```python
from build123d import *

# Parameters (mm, degrees)
F1_DEPTH = 1000


with BuildPart() as f1:
    # F0 (on Front) → F1 (new body)
    with BuildSketch(Plane.XZ):
        with BuildLine():
            Line((-72.4, 558.240645), (-72.4, 541.240645))
            Line((-72.4, 541.240645), (82, 541.240645))
            Line((82, 541.240645), (82, 558.240645))
            Line((82, 558.240645), (19.8, 558.240645))
            ThreePointArc((19.8, 558.240645), (12.587511, 561.228156), (9.6, 568.440645))
            Line((9.6, 568.440645), (9.6, 976.040645))
            ThreePointArc((9.6, 976.040645), (12.587511, 983.253134), (19.8, 986.240645))
            Line((19.8, 986.240645), (82, 986.240645))
            Line((82, 986.240645), (82, 1003.240645))
            Line((82, 1003.240645), (-72.4, 1003.240645))
            Line((-72.4, 1003.240645), (-72.4, 986.240645))
            Line((-72.4, 986.240645), (-10.2, 986.240645))
            ThreePointArc((-10.2, 986.240645), (-2.987511, 983.253134), (0, 976.040645))
            Line((0, 976.040645), (0, 568.440645))
            ThreePointArc((0, 568.440645), (-2.987511, 561.228156), (-10.2, 558.240645))
            Line((-10.2, 558.240645), (-72.4, 558.240645))
        make_face()
    extrude(amount=-F1_DEPTH)


solid = f1.part
```
Work out the finished part from the listing and answer in its coordinate system (mm). A direction names the side the tool comes from. Give positions to 0.01 mm unless a question says otherwise; leave off trailing zeros. Order: outer loops, then holes, each group sorted by start corner. A loop starts at its lowest first (then second) coordinate and runs counter-clockwise, first axis right, second up. Notation, with made-up numbers: (-26.75, 57) -> (26.25, 57) arc R23 ccw to (26.25, 89) -> close; hole circle Ø1 at (52.25, 58.5). An arc over 180 degrees is marked (long way). Answer as CSV lines item,"result". Start each with the question number.
(1) Section C-C, the plane z = 959 is taken. Write down the section's boundary in (x, y).
(2) Consider line 1 along Z through (x, y) = (64, 953); line 2 along Z through (x, y) = (-9.5, 335.5); line 3 along X through (y, z) = (649, 893). Determine where each line is inside the solid, lowest interval first.
(3) Which of the six approach directions +Z, -Z, +X, -X, +Y, -Y give full straight-line access (tool end or side, diameter ignored) to faces 1 (the flat face through (-41, 493, 558.241)), 2 (the flat face through (51, 493, 558.241)), 3 (the flat face through (6, 493, 1003.241))?
(4) Section B-B, the plane y = 158.5 is taken. Write down the section's boundary in (x, z).
(5) For a pull along Z with two mould halves and no side action, classify faces 4 (the flat face through (-72.4, 493, 550)), 5 (the flat face through (50, 493, 986.241)), 6 (the flat face through (4, 493, 541.241)) as released by +Z, released by -Z, zero draft, split by the parting line, or undercut.
(6) Each of these flat-tipped pins is pushed along its axis until it touches: pin 1 Ø10 at (y, z) = (124, 629) entering from -X; pin 2 Ø6 at (x, z) = (3, 786.5) entering from -Y. Where does it stop, or does it pass through?
(7) Section A-A, the plane x = -22 is taken. Write down the section's boundary in (y, z), plus the area to 3 significant figures.
Entries:
1,outline,"(0, 0) -> (9.6, 0) -> (9.6, 1000) -> (0, 1000) -> close"
2,line 1,"541.24 to 558.24, 986.24 to 1003.24"
2,line 2,"541.24 to 558.26, 986.22 to 1003.24"
2,line 3,"0 to 9.6"
3,face 1,"-X, +Y, -Y"
3,face 2,"+X, +Y, -Y"
3,face 3,"+Z, +X, -X, +Y, -Y"
4,outline,"(-72.4, 541.24) -> (82, 541.24) -> (82, 558.24) -> (19.8, 558.24) arc R10.2 cw to (9.6, 568.44) -> (9.6, 976.04) arc R10.2 cw to (19.8, 986.24) -> (82, 986.24) -> (82, 1003.24) -> (-72.4, 1003.24) -> (-72.4, 986.24) -> (-10.2, 986.24) arc R10.2 cw to (0, 976.04) -> (0, 568.44) arc R10.2 cw to (-10.2, 558.24) -> (-72.4, 558.24) -> close"
5,face 4,"zero draft"
5,face 5,"undercut"
5,face 6,"released by -Z"
6,pin 1,"x = 0"
6,pin 2,"y = 0"
7,outline,"(0, 541.24) -> (1000, 541.24) -> (1000, 558.24) -> (0, 558.24) -> close; (0, 986.24) -> (1000, 986.24) -> (1000, 1003.24) -> (0, 1003.24) -> close"
7,area,"34,000 mm²"
